Autodesk Inventor part; units mm, degrees
ref_plane "YZ Plane" through (0, 0, 0) normal (1, 0, 0) x (0, 1, 0)
ref_plane "XZ Plane" through (0, 0, 0) normal (0, 1, 0) x (-1, 0, 0)
ref_plane "XY Plane" through (0, 0, 0) normal (0, 0, 1) x (1, 0, 0)
sketch "Sketch1" plane through (0, 0, 0) normal (0, 0, 1) x (1, 0, 0)
  line L0 (-5.715, -10.16) -> (5.715, -10.16)
  line L1 (5.715, -10.16) -> (5.715, 10.16)
  line L2 (5.715, 10.16) -> (-5.715, 10.16)
  line L3 (-5.715, 10.16) -> (-5.715, -10.16)
  line L4 (-5.715, -10.16) -> (5.715, 10.16) construction
  line L5 (5.715, -10.16) -> (-5.715, 10.16) construction
  point P0 (0, 0)
  dimension "d0" = 20.32
  dimension "d1" = 11.43
extrude "Extrusion1" add sketch "Sketch1" along normal blind 6.35
sketch "Sketch2" plane through (0, 0, 6.35) normal (0, 0, 1) x (1, 0, 0)
  line L0 (-5.715, 10.16) -> (-5.715, -10.16)
  line L1 (-5.715, -10.16) -> (5.715, -10.16)
  point P0 (0, 0)
  point P1 (0, -5.1562)
  dimension "d5" = 5.0038
  dimension "d22" = 5.715
hole "Hole1" at (0, -5.1562, 6.35) direction (0, 0, -1) diameter 3 end through all
sketch "Sketch3" plane through (0, 0, 6.35) normal (0, 0, 1) x (1, 0, 0)
  line L0 (-5.715, -10.16) -> (5.715, -10.16)
  line L1 (5.715, -10.16) -> (5.715, 10.16)
  point P0 (0, 0)
  point P1 (0, 4.848)
  dimension "d13" = 15.008
  dimension "d14" = 5.715
hole "Hole2" at (0, 4.848, 6.35) direction (0, 0, -1) diameter 6 end through all countersink diameter 8.4 countersink angle 45
fillet "Fillet1" radius 1.5875 4 edges at (5.715, 10.16, 3.175) (-5.715, 10.16, 3.175) (5.715, -10.16, 3.175) (-5.715, -10.16, 3.175)
sketch "Sketch4" plane through (0, 0, 0) normal (0, 0, -1) x (-1, 0, 0)
  circle A0 centre (0, 4.848) radius 3
  circle A1 centre (0, 4.848) radius 3.9
  circle A2 centre (0, 4.848) radius 3 construction
  point P0 (0, 0)
  dimension "d27" = 7.8
extrude "Extrusion2" add sketch "Sketch4" along normal blind 1.27
chamfer "Chamfer2" distance 0.635 angle 45 3 edges at (0, -3.6562, 0) (0, -3.6562, 6.35) (3.9, 4.848, -1.27)
properties part number "beam_break_spacer" material "Aluminum 6061"
Design review of the part built by this model. Coordinates are the model's own, in mm. A direction names the side the tool comes from. Round coordinates to 2 decimals unless told otherwise and drop trailing zeros. Write each loop counter-clockwise with the first axis right and the second up, starting at its lowest first coordinate (ties: lowest second). Pieces come first, ordered by that corner, then holes. Notation, with made-up numbers: (-33.75, -1) -> (-3.75, -1) arc R20 ccw to (-3.75, 8) -> close; hole circle Ø10 at (-30, 87). An arc over 180 degrees is marked (long way). Answer in a Markdown table with one row per item.
Q1. Clearance check with flat-ended pins moving along their axes: pin 1 Ø3.5 at (x, y) = (0, -5.16) entering from -Z; pin 2 Ø1 at (x, y) = (-3, -0.5) entering from -Z. State where each tip first meets the part, or that it passes through.
The answers:
| item | result |
|---|---|
| pin 1 | z = 0.38 |
| pin 2 | z = 0 |
Q2. Take a section at C-C, the plane z = 6. State the section outline as (x, y) points (1 decimal), then the cut area to 3 significant figures.
The answers:
| item | result |
|---|---|
| outline | (-5.7, -8.6) arc R1.6 ccw to (-4.1, -10.2) -> (4.1, -10.2) arc R1.6 ccw to (5.7, -8.6) -> (5.7, 8.6) arc R1.6 ccw to (4.1, 10.2) -> (-4.1, 10.2) arc R1.6 ccw to (-5.7, 8.6) -> close; hole circle Ø8.1 at (0, 4.8); hole circle Ø3.6 at (0, -5.2) |
| area | 168 mm² |
Q3. Draft analysis for pull direction Y (two halves, no side actions). For faces 3 (the face through (0, -10.16, 3)), 4 (the face through (-2.645, 3.433, 1.058)), 5 (the face through (0, 0, 0)), state which applies: +Y half, -Y half, draft (parallel to the pull), parting line (faces both ways), or undercut.
The answers:
| item | result |
|---|---|
| face 3 | -Y half |
| face 4 | undercut |
| face 5 | draft |
Q4. For faces 1 (the face through (3.095, 7.221, -0.313)), 2 (the face through (-2.728, 3.429, 3.634)), list the 3-axis set-ups (+Z, -Z, +X, -X, +Y, -Y) from which the entire face can be reached by the end or side of a thin tool; tool diameter is ignored.
The answers:
| item | result |
|---|---|
| face 1 | -Z |
| face 2 | +Z |
Q5. Take a section at B-B, the plane z = 1.75. State the section outline as (x, y) points (1 decimal), then the cut area to 3 significant figures.
The answers:
| item | result |
|---|---|
| outline | (-5.7, -8.6) arc R1.6 ccw to (-4.1, -10.2) -> (4.1, -10.2) arc R1.6 ccw to (5.7, -8.6) -> (5.7, 8.6) arc R1.6 ccw to (4.1, 10.2) -> (-4.1, 10.2) arc R1.6 ccw to (-5.7, 8.6) -> close; hole circle Ø6 at (0, 4.8); hole circle Ø3 at (0, -5.2) |
| area | 195 mm² |
Q6. Take a section at A-A, the plane x = 0. State the section outline as (y, z) points (3 decimals).
The answers:
| item | result |
|---|---|
| outline | (-10.16, 0) -> (-7.291, 0) -> (-6.656, 0.635) -> (-6.656, 5.715) -> (-7.291, 6.35) -> (-10.16, 6.35) -> close; (-3.656, 0.635) -> (-3.021, 0) -> (0.948, 0) -> (0.948, -0.635) -> (1.583, -1.27) -> (1.848, -1.27) -> (1.848, 3.453) -> (0.648, 6.35) -> (-3.021, 6.35) -> (-3.656, 5.715) -> close; (7.848, -1.27) -> (8.113, -1.27) -> (8.748, -0.635) -> (8.748, 0) -> (10.16, 0) -> (10.16, 6.35) -> (9.048, 6.35) -> (7.848, 3.453) -> close |
Q7. To check wall thickness, follow L1, parallel to Y at x = 0, z = 2.3; L2, parallel to X at y = 5, z = 1.5 (3 decimals); L3, parallel to Y at x = -0.5, z = 1.25. State the ranges of each line that lie inside material, in increasing order. Write a range as [from, to].
The answers:
| item | result |
|---|---|
| L1 | [-10.16, -6.66], [-3.66, 1.85], [7.85, 10.16] |
| L2 | [-5.715, -2.996], [2.996, 5.715] |
| L3 | [-10.16, -6.57], [-3.74, 1.89], [7.81, 10.16] |
Q8. Take a section at D-D, the plane x = -1.25. Count the separate pieces of the cut face and the enclosed holes in it, then the cut area to 3 significant figures.
The answers:
| item | result |
|---|---|
| separate pieces | 3 |
| enclosed holes | 0 |
| area | 80.9 mm² |
